```python
from build123d import *

# Parameters (mm, degrees)
BOSS_EXTRUDE1_DEPTH            = 40
F_13_0_13_DIAMETER_HOLE1_D     = 13
F_13_0_13_DIAMETER_HOLE1_DEPTH = 29
CUT_EXTRUDE8_DEPTH             = 16
SKETCH14_R                     = 6.35
SKETCH14_R_2                   = 5.502637429
CUT_EXTRUDE9_DEPTH             = 10
CUT_EXTRUDE10_DEPTH            = 10


with BuildPart() as part:
    # Sketch1 → Boss-Extrude1 (new body)
    with BuildSketch(Plane(origin=(0, 20, 0), x_dir=(1, 0, 0), z_dir=(0, 1, 0))):
        with BuildLine():
            Line((563.96485174, 507.513718698), (563.96485174, 562.736423486))
            Line((563.96485174, 562.736423486), (554.690781869, 562.894803628))
            ThreePointArc((554.690781869, 562.894803628), (545.704943994, 565.795150829), (539.853906856, 573.206133263))
            Line((539.853906856, 573.206133263), (522.524343645, 610.429990226))
            ThreePointArc((522.524343645, 610.429990226), (512.649800976, 621.543175495), (497.931198247, 623.634159339))
            Line((497.931198247, 623.634159339), (399.830947056, 608.608698386))
            ThreePointArc((399.830947056, 608.608698386), (385.610832142, 608.137408426), (371.923585817, 612.02238853))
            Line((371.923585817, 612.02238853), (95.310746964, 771.494097008))
            add(Edge.make_bspline(
                [(60.287007155, 752.902507236), (59.408683029, 762.769524202), (58.560960325, 776.204376236), (76.94287295, 783.298520304), (86.753146937, 776.493697586), (95.310746964, 771.494097008)],
                knots=[0, 0, 0, 0, 0.5, 0.5, 1, 1, 1, 1], degree=3))
            ThreePointArc((60.287007155, 752.902507236), (112.407005996, 551.803928099), (202.762947005, 364.739937083))
            ThreePointArc((202.762947005, 364.739937083), (207.132055784, 361.391783138), (212.632195034, 361.173346422))
            Line((212.632195034, 361.173346422), (367.65464082, 417.084401042))
            ThreePointArc((367.65464082, 417.084401042), (380.966681082, 418.419109504), (394.090964942, 415.82198883))
            Line((394.090964942, 415.82198883), (660.231475403, 329.574923038))
            ThreePointArc((660.231475403, 329.574923038), (670.878462163, 333.606992627), (669.266978502, 344.877264703))
            Line((669.266978502, 344.877264703), (553.73117364, 453.239940989))
            ThreePointArc((553.73117364, 453.239940989), (543.342125743, 483.300566911), (563.96485174, 507.513718698))
        make_face()
    extrude(amount=-BOSS_EXTRUDE1_DEPTH)

    # Ø13.0 (13) Diameter Hole1
    with Locations(Plane(origin=(0, 20, 0), x_dir=(1, 0, 0), z_dir=(0, 1, 0))):
        with Locations((274.335910331, 496.233480955), (274.335910331, 579.213058938)):
            Hole(F_13_0_13_DIAMETER_HOLE1_D / 2, depth=F_13_0_13_DIAMETER_HOLE1_DEPTH)

    # Sketch13 → Cut-Extrude8 (cut)
    with BuildSketch(Plane(origin=(0, 20, 0), x_dir=(1, 0, 0), z_dir=(0, 1, 0))):
        with BuildLine():
            Line((563.96485174, 563.125071092), (496.273234513, 563.125071092))
            ThreePointArc((496.273234513, 563.125071092), (492.20587406, 561.651450789), (490.026307291, 557.914544776))
            ThreePointArc((490.026307291, 557.914544776), (487.96485174, 535.125071092), (490.026307291, 512.335597408))
            ThreePointArc((490.026307291, 512.335597408), (492.20587406, 508.598691395), (496.273234513, 507.125071092))
            Line((496.273234513, 507.125071092), (563.96485174, 507.125071092))
            Line((563.96485174, 507.125071092), (563.96485174, 563.125071092))
        make_face()
    extrude(amount=-CUT_EXTRUDE8_DEPTH, mode=Mode.SUBTRACT)

    # Sketch14 → Cut-Extrude9 (cut)
    with BuildSketch(Plane(origin=(0, 20, 0), x_dir=(1, 0, 0), z_dir=(0, 1, 0))):
        with Locations(Location((303.81485174, 498.131405852, 0), (0, 0, 270))):
            Circle(SKETCH14_R)
        with Locations(Location((298.641153596, 572.118736332, 0), (0, 0, 270))):
            Circle(SKETCH14_R_2)
    extrude(amount=-CUT_EXTRUDE9_DEPTH, mode=Mode.SUBTRACT)

    # Sketch17 → Cut-Extrude10 (cut)
    with BuildSketch(Plane(origin=(0, 20, 0), x_dir=(1, 0, 0), z_dir=(0, 1, 0))):
        with BuildLine():
            Line((481.61485174, 499.042173829), (481.61485174, 571.207968354))
            ThreePointArc((481.61485174, 571.207968354), (473.296544122, 580.314612527), (463.475969831, 572.852606745))
            Line((463.475969831, 572.852606745), (457.73885174, 541.475071092))
            Line((457.73885174, 541.475071092), (457.73885174, 528.775071092))
            Line((457.73885174, 528.775071092), (463.475969831, 497.397535439))
            ThreePointArc((463.475969831, 497.397535439), (473.296544122, 489.935529657), (481.61485174, 499.042173829))
        make_face()
        with BuildLine():
            Line((420.65485174, 499.042173829), (420.65485174, 571.207968354))
            ThreePointArc((420.65485174, 571.207968354), (412.336544122, 580.314612527), (402.515969831, 572.852606745))
            Line((402.515969831, 572.852606745), (396.77885174, 541.475071092))
            Line((396.77885174, 541.475071092), (396.77885174, 528.775071092))
            Line((396.77885174, 528.775071092), (402.515969831, 497.397535439))
            ThreePointArc((402.515969831, 497.397535439), (412.336544122, 489.935529657), (420.65485174, 499.042173829))
        make_face()
        with BuildLine():
            Line((357.072977222, 497.929527206), (372.077089581, 568.518325976))
            ThreePointArc((372.077089581, 568.518325976), (365.83393473, 579.155441526), (354.67652531, 573.898310679))
            Line((354.67652531, 573.898310679), (342.541020523, 544.399263386))
            Line((342.541020523, 544.399263386), (339.90054205, 531.976788856))
            Line((339.90054205, 531.976788856), (338.988533854, 500.092113718))
            ThreePointArc((338.988533854, 500.092113718), (347.043066796, 490.751358459), (357.072977222, 497.929527206))
        make_face()
    extrude(amount=-CUT_EXTRUDE10_DEPTH, mode=Mode.SUBTRACT)


solid = part.part
```
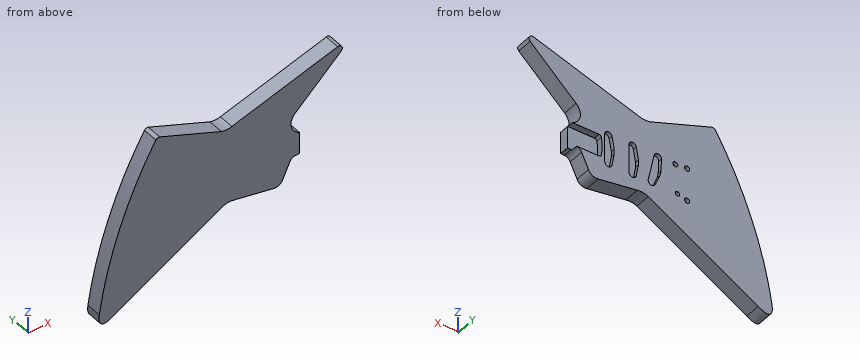
Could you check a few things on this model? Use its own coordinates, in mm. Coordinates: 2 decimals unless noted, no trailing zeros. Order: outer loops, then holes, each group sorted by start corner. A loop starts at its lowest first (then second) coordinate and runs counter-clockwise, first axis right, second up. Notation, with made-up numbers: M 40.5,-21 L 89.5,-21 A7 ccw 89.5,-11 Z; hole C 46.5,63.25 d9. An arc over 180 degrees is marked long. Use one line per item in the form item = value. Start each with the question number.
1. Suppose I cut it at C-C on x = 254. Write out the boundary of the cut face in (y, z).
2. Suppose I cut it at A-A on x = 474.5. Write out the boundary of the cut face in (y, z), then the cut area to 3 significant figures.
3. Please list where these lines run through material, in increasing order: line 1 (Y direction, x = 409, z = -519); line 2 (Z direction, x = 547.5, y = 13); line 3 (X direction, y = 8.5, z = -763).
4. For pin 1 (3.5 mm diameter, centred on x = 298.5, z = -570, fed in from +Y); pin 2 (4 mm diameter, centred on x = 275, z = -495, fed in from +Y); pin 3 (8 mm diameter, centred on y = -10, z = -381.5, fed in from +X); pin 4 (12.5 mm diameter, centred on x = 298.64, z = -572.12, fed in from +Y), each with a flat end and sliding along its axis, tell me the tip position at first contact or that it passes through.
5. Suppose I cut it at B-B on z = -642. Write out the boundary of the cut face in (x, y), then the cut area to 4 significant figures.
Geometry says:
q1.outline = M -20,-680.01 L 20,-680.01 L 20,-376.09 L -20,-376.09 Z
q2.outline = M -20,-620.05 L 20,-620.05 L 20,-580.12 L 10,-580.12 L 10,-490.13 L 20,-490.13 L 20,-389.76 L -20,-389.76 Z
q2.area = 8,310 mm^2
q3.line_1 = -20 to 10
q3.line_2 = -564.71 to -563.13, -507.13 to -494.09, -460.63 to -366.11
q3.line_3 = 59.78 to 110.04
q4.pin_1 = 10
q4.pin_2 = -9
q4.pin_3 = 634.48
q4.pin_4 = 20
q5.outline = M 83.8,-20 L 319.93,-20 L 319.93,20 L 83.8,20 Z
q5.area = 9,445 mm^2
